Work out the finished part from the listing and answer in its coordinate system (mm). Coordinates: 2 decimals unless noted, no trailing zeros. Use one line per item in the form item = value.
Autodesk Inventor part; units mm, degrees
ref_plane "YZ Plane" through (0, 0, 0) normal (1, 0, 0) x (0, 1, 0)
ref_plane "XZ Plane" through (0, 0, 0) normal (0, 1, 0) x (-1, 0, 0)
ref_plane "XY Plane" through (0, 0, 0) normal (0, 0, 1) x (1, 0, 0)
sketch "Sketch1" plane through (0, 0, 0) normal (0, 0, 1) x (1, 0, 0)
  line L0 (0, 0) -> (0, 22.3)
  line L1 (0, 0) -> (9, 0)
  spline S0 degree 4 poles (0, 22.3) (5.9332, 19.4872) (8.095, 9.9218) (8.9717, 6.9333) (9, 0) knots 0 0 0 0 0 1 1 1 1 1
  point P0 (7.5, 11.15)
  point P1 (4.8515, 17.3878)
  point P2 (8.6406, 5.8553)
revolve "Revolution1" add sketch "Sketch1" angle 360 about axis through (0, 0, 0) along (0, 1, 0)
sketch "Sketch2" plane through (0, 0, 0) normal (0, 0, 1) x (1, 0, 0)
  circle A0 centre (0, 15) radius 2
extrude "Extrusion1" cut sketch "Sketch2" along normal mid plane 15
sketch "Sketch3" plane through (0, 0, 0) normal (0, -1, 0) x (1, 0, 0)
  circle A0 centre (0, 0) radius 2.5
  dimension "d8" = 5
extrude "Extrusion3" cut sketch "Sketch3" against normal blind 13
chamfer "Chamfer1" distance 0.5 angle 45 1 edges at (-2.5, 0, 0)
thread "Thread6"
properties part number "nose-over"
(1) The mould has two halves that part along X. Classify faces 1 (the cylindrical face through (-0.54, 6.66, -2.44)), 2 (the flat face through (0, 0, 4)): released by +X, released by -X, zero draft, split by the parting line, or undercut.
Data:
face_1 = undercut
face_2 = zero draft
(2) Straight lines are drawn through the part: line 1 along X through (y, z) = (12.25, 2); line 2 along Z through (x, y) = (-1.5, 9.5); line 3 along Z through (x, y) = (0, 10.25). For each, find the intervals that lie inside material, in ascending order.
Data:
line_1 = -6.87 to -1.5, 1.5 to 6.87
line_2 = -7.81 to -2, 2 to 7.81
line_3 = -7.76 to -2.5, 2.5 to 7.76
(3) Each of these flat-tipped pins is pushed along its axis until it touches: P1, Ø4, axis at x = 5.5, z = -2, coming from the -Y side; P2, Ø1.3, axis at x = 1, z = 0, coming from the -Y side; P3, Ø10, axis at x = 4, y = 14, coming from the -Z side; P4, Ø8, axis at x = 5.5, z = 6, coming from the +Y side. Where does it stop, or does it pass through?
Data:
P1 = 0
P2 = 13
P3 = -7.77
P4 = 18.5
